```python
from build123d import *

# Parameters (mm, degrees)
SKETCH2_W           = 140
SKETCH2_H           = 150
BOSS_EXTRUDE1_DEPTH = 240
SKETCH3_R           = 65
BOSS_EXTRUDE2_DEPTH = 50
SKETCH4_R           = 70
BOSS_EXTRUDE3_DEPTH = 10
SKETCH5_R           = 50
BOSS_EXTRUDE4_DEPTH = 80
FILLET1_R           = 10
SKETCH6_R           = 65
BOSS_EXTRUDE5_DEPTH = 20
BOSS_EXTRUDE6_DEPTH = 70
CUT_EXTRUDE1_DEPTH  = 50
BOSS_EXTRUDE7_REACH = 650.407
SKETCH9_R           = 50


with BuildPart() as part:
    # Sketch2 → Boss-Extrude1 (new body)
    with BuildSketch(Plane(origin=(0, 0, 0), x_dir=(0, 0, -1), z_dir=(1, 0, 0))):
        Rectangle(SKETCH2_W, SKETCH2_H)
    extrude(amount=BOSS_EXTRUDE1_DEPTH)

    # Sketch3 → Boss-Extrude2 (add)
    with BuildSketch(Plane(origin=(240, 0, 0), x_dir=(0, 0, -1), z_dir=(1, 0, 0))):
        Circle(SKETCH3_R)
    extrude(amount=BOSS_EXTRUDE2_DEPTH)

    # Sketch4 → Boss-Extrude3 (add)
    with BuildSketch(Plane(origin=(290, 0, 0), x_dir=(0, 0, -1), z_dir=(1, 0, 0))):
        Circle(SKETCH4_R)
    extrude(amount=BOSS_EXTRUDE3_DEPTH)

    # Sketch5 → Boss-Extrude4 (add, symmetric)
    with BuildSketch(Plane.XY):
        with BuildLine():
            Line((170.044787747, -145), (170.044787747, -75))
            Line((170.044787747, -75), (0, -75))
            Line((0, -75), (16.218764607, -158.438310593))
            ThreePointArc((16.218764607, -158.438310593), (99.289534096, -222.205947936), (170.044787747, -145))
        make_face()
        with Locations((92.544787747, -145)):
            Circle(SKETCH5_R, mode=Mode.SUBTRACT)
    extrude(amount=BOSS_EXTRUDE4_DEPTH, both=True)

    # Fillet1
    fillet1_edges = [part.edges().sort_by_distance(p)[0] for p in [
        (85.022393874, -75, -70),
        (85.022393874, -75, 70),
    ]]
    fillet(fillet1_edges, radius=FILLET1_R - 0.0001)  # a hair under: the kernel refuses the full size

    # Sketch6 → Boss-Extrude5 (add)
    with BuildSketch(Plane(origin=(300, 0, 0), x_dir=(0, 0, -1), z_dir=(1, 0, 0))):
        Circle(SKETCH6_R)
    extrude(amount=BOSS_EXTRUDE5_DEPTH)

    # Sketch7 → Boss-Extrude6 (add, symmetric)
    with BuildSketch(Plane.XY):
        with BuildLine():
            Line((520, -75), (320, -75))
            Line((320, -75), (320, 75))
            Line((320, 75), (520, 75))
            ThreePointArc((520, 75), (595, 0), (520, -75))
        make_face()
    extrude(amount=BOSS_EXTRUDE6_DEPTH, both=True)

    # Sketch8 → Cut-Extrude1 (cut, symmetric)
    with BuildSketch(Plane.XY):
        with BuildLine():
            Line((520, 75), (420, 75))
            Line((420, 75), (420, -75))
            Line((420, -75), (520, -75))
            ThreePointArc((520, -75), (595, 0), (520, 75))
        make_face()
    extrude(amount=CUT_EXTRUDE1_DEPTH, both=True, mode=Mode.SUBTRACT)

    # Sketch9 → Boss-Extrude7 (add, up to next)
    with BuildSketch(Plane.XY.offset(-50), mode=Mode.PRIVATE) as boss_extrude7_sk1:
        with Locations((520, 0)):
            Circle(SKETCH9_R)
    boss_extrude7_tool1 = extrude(boss_extrude7_sk1.sketch, amount=BOSS_EXTRUDE7_REACH, mode=Mode.PRIVATE) - part.part
    add(boss_extrude7_tool1.solids().sort_by_distance((520, 0, -50))[0])


solid = part.part
```
Could you check a few things on this model? Use its own coordinates, in mm. A direction names the side the tool comes from. Coordinates: 2 decimals unless noted, no trailing zeros. Order: outer loops, then holes, each group sorted by start corner. A loop starts at its lowest first (then second) coordinate and runs counter-clockwise, first axis right, second up. Notation, with made-up numbers: M 70.5,49.5 L 84.5,49.5 A21 cw 84.5,55.5 Z; hole C -7,7 d9. An arc over 180 degrees is marked long. Use a Markdown table: item, result. Add a question column.
Q1. We'd pull the mould along X, two halves only. Please class faces 1 (the flat face through (65, -99, 80)), 2 (the flat face through (467, 1, -50)), 3 (the flat face through (7.996, -116.135, 1.12)): pulls with the +X half, pulls with the -X half, needs draft (parallel to the pull), parting line crosses it, or undercut.
Q2. If I drill on L1, parallel to X at y = 61, z = -43.5; L2, parallel to Y at x = 174, z = -36; L3, parallel to Z at x = 143, y = -66, over which ranges is the centre line in solid material (lowest first)?
Q3. I want a section at A-A on z = 0. List the corners of the cut face in (x, y) for me, then the cut area to 3 significant figures.
Q4. I'm going to push flat-ended pins straight in: pin 1 (3 mm diameter, centred on y = -175, z = 5, fed in from +X); pin 2 (12 mm diameter, centred on x = 128, z = -62, fed in from -Y). Where does each tip first touch, or does it pass through?
Q5. I want a section at B-B on y = 0. List the corners of the cut face in (x, z) for me, then the cut area to 3 significant figures.
Q6. Which directions (+Z, -Z, +X, -X, +Y, -Y) give clear straight access to the entire face, cutting with the end or side of a thin tool? Please do faces 4 (the flat face through (290, -61.9, -20.4)), 5 (the flat face through (205, -75, 1)), 6 (the flat face through (0, 1, 1)).
Q7. I want a section at D-D on y = -171. List the corners of the cut face in (x, z) for me, then the cut area to 3 significant figures.
Checked values:
| question | item | result |
|---|---|---|
| 1 | face 1 | needs draft |
| 1 | face 2 | undercut |
| 1 | face 3 | pulls with the -X half |
| 2 | L1 | 0 to 240, 320 to 420 |
| 2 | L2 | -75 to 75 |
| 2 | L3 | -70.05 to 70.05 |
| 3 | outline | M 0,-75 L 16.22,-158.44 A77.5 ccw 170.04,-145 L 170.04,-75 L 240,-75 L 240,-65 L 290,-65 L 290,-70 L 300,-70 L 300,-65 L 320,-65 L 320,-75 L 420,-75 L 420,75 L 320,75 L 320,65 L 300,65 L 300,70 L 290,70 L 290,65 L 240,65 L 240,75 L 0,75 Z; C 520,0 d100; hole C 92.54,-145 d100 |
| 3 | area | 82,400 mm² |
| 4 | pin 1 | x = 164.61 |
| 4 | pin 2 | y = -216.68 |
| 5 | outline | M 0,-70 L 240,-70 L 240,-65 L 290,-65 L 290,-70 L 300,-70 L 300,-65 L 320,-65 L 320,-70 L 595,-70 L 595,-50 L 570,-50 L 570,50 L 595,50 L 595,70 L 320,70 L 320,65 L 300,65 L 300,70 L 290,70 L 290,65 L 240,65 L 240,70 L 0,70 Z; hole M 420,-50 L 470,-50 L 470,50 L 420,50 Z |
| 5 | area | 75,100 mm² |
| 6 | face 4 | none |
| 6 | face 5 | +Z, -Z, +X, -Y |
| 6 | face 6 | +Z, -Z, -X, +Y, -Y |
| 7 | outline | M 19.54,-80 L 49.84,-80 L 49.84,80 L 19.54,80 Z; M 135.25,-80 L 165.55,-80 L 165.55,80 L 135.25,80 Z |
| 7 | area | 9,700 mm² |
